Check sheet for the modelled part. Datum: model origin and axes. Units: mm. Face numbers are marked on the shaded views. Give positions to 0.01 mm unless a question says otherwise; leave off trailing zeros. Loops run counter-clockwise (first coordinate to the right, second up) from the corner with the lowest first, then second, coordinate; pieces in that order, holes last. Notation, with made-up numbers: (-15, 16) -> (-10, 16) arc R28 ccw to (-10, 49) -> close; hole circle Ø5 at (73, 33.25). An arc over 180 degrees is marked (long way). Write each question's results on one line, items separated by ' | '. Start each with the question number.
Item 1: Cross-section at C-C on z = 7.5. Enter the section's corners in (x, y), then the cut area to 3 significant figures.
Item 2: Gauge pin test, flat ends, axial feed: pin 1 Ø4 at (y, z) = (-8.5, 3.5) entering from -X; pin 2 Ø4 at (x, y) = (4, -2.5) entering from -Z; pin 3 Ø2 at (x, z) = (7.5, 6.5) entering from +Y; pin 4 Ø3 at (x, z) = (4, 3) entering from +Y. Record the tip position at first contact, or that the pin passes through.
Item 3: Mould release check, pull along X, two halves, no side actions. Record for the marked faces 1, 2, 3 and 4: pulls with the +X half, pulls with the -X half, needs draft (parallel to the pull), parting line crosses it, or undercut.
Item 4: Cross-section at A-A on y = 0. Enter the section's corners in (x, z) (3 decimals), then the cut area to 3 significant figures.
Item 5: Scan lines: line 1 along Y through (x, z) = (0, 6.5); line 2 along Y through (x, z) = (-5.25, 3.75); line 3 along X through (y, z) = (-3, 1.75). Record each from-to range of solid material in increasing order.
Item 6: Cross-section at B-B on x = 0. Enter the section's corners in (y, z) (3 decimals).
Item 7: Cross-section at D-D on y = -9. Enter the section's corners in (x, z) (3 decimals), then the cut area to 3 significant figures.
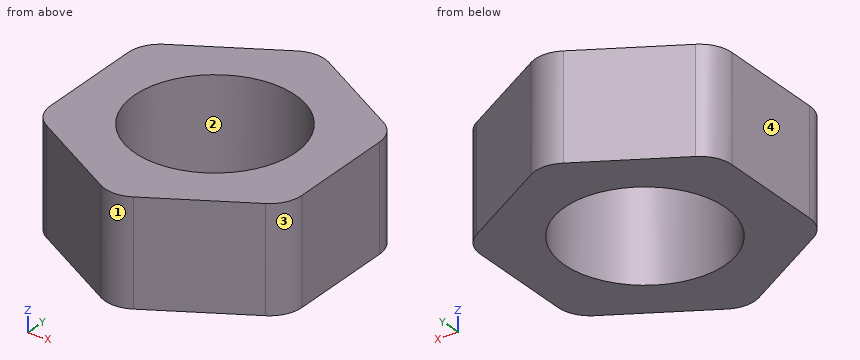
from build123d import *

# Parameters (mm, degrees)
F0_R     = 6.35
F1_DEPTH = 8.255
F2_R     = 2.54


with BuildPart() as f1:
    # F0 (on Top) → F1 (new body)
    with BuildSketch(Plane.XY):
        Polygon((9.89867, 5.715), (0, 11.43), (-9.89867, 5.715), (-9.89867, -5.715), (0, -11.43), (9.89867, -5.715), align=None)
        Circle(F0_R, mode=Mode.SUBTRACT)
    extrude(amount=F1_DEPTH)

    # F2
    f2_edges = [f1.edges().sort_by_distance(p)[0] for p in [
        (-9.89867, -5.715, 4.1275),
        (0, -11.43, 4.1275),
        (9.89867, -5.715, 4.1275),
        (9.89867, 5.715, 4.1275),
        (0, 11.43, 4.1275),
        (-9.89867, 5.715, 4.1275),
    ]]
    fillet(f2_edges, radius=F2_R)


solid = f1.part
Answer sheet:
1) outline: (-9.9, -4.25) arc R2.54 ccw to (-8.63, -6.45) -> (-1.27, -10.7) arc R2.54 ccw to (1.27, -10.7) -> (8.63, -6.45) arc R2.54 ccw to (9.9, -4.25) -> (9.9, 4.25) arc R2.54 ccw to (8.63, 6.45) -> (1.27, 10.7) arc R2.54 ccw to (-1.27, 10.7) -> (-8.63, 6.45) arc R2.54 ccw to (-9.9, 4.25) -> close; hole circle Ø12.7 at (0, 0) | area: 211 mm²
2) pin 1: stops at x = -8.54 | pin 2: stops at z = 0 | pin 3: stops at y = 7.68 | pin 4: stops at y = 9.99
3) face 1: parting line crosses it | face 2: undercut | face 3: pulls with the +X half | face 4: pulls with the -X half
4) outline: (-9.899, 0) -> (-6.35, 0) -> (-6.35, 8.255) -> (-9.899, 8.255) -> close; (6.35, 0) -> (9.899, 0) -> (9.899, 8.255) -> (6.35, 8.255) -> close | area: 58.6 mm²
5) line 1: y = -11.04 to -6.35, 6.35 to 11.04 | line 2: y = -8.4 to -3.57, 3.57 to 8.4 | line 3: x = -9.9 to -5.6, 5.6 to 9.9
6) outline: (-11.037, 0) -> (-6.35, 0) -> (-6.35, 8.255) -> (-11.037, 8.255) -> close; (6.35, 0) -> (11.037, 0) -> (11.037, 8.255) -> (6.35, 8.255) -> close
7) outline: (-4.209, 0) -> (4.209, 0) -> (4.209, 8.255) -> (-4.209, 8.255) -> close | area: 69.5 mm²
